Autodesk Inventor part; units mm, degrees
ref_plane "Work Plane1" through (277, 0, 0) normal (1, 0, 0) x (0, 1, 0)
ref_plane "Work Plane2" through (0, 40, 0) normal (0, 1, 0) x (-1, 0, 0)
ref_plane "XY Plane" through (0, 0, 0) normal (0, 0, 1) x (1, 0, 0)
sketch "Sketch1" plane through (0, 0, 0) normal (0, 0, 1) x (1, 0, 0)
  line L0 (955, 0) -> (955, 80)
  line L1 (0, 80) -> (0, 0)
  line L2 (277, 0) -> (277, 20)
  line L3 (277, 20) -> (733, 20)
  line L4 (733, 20) -> (733, 0)
  line L5 (277, 80) -> (277, 60)
  line L6 (277, 60) -> (733, 60)
  line L7 (733, 60) -> (733, 80)
  line L8 (0, 80) -> (955, 80)
  line L9 (427, 0) -> (427, 20)
  line L10 (583, 0) -> (583, 20)
  line L11 (0, 0) -> (955, 0)
  line L12 (277, 0) -> (733, 0)
  line L13 (733, 80) -> (277, 80)
  dimension "d0" = 955
  dimension "d1" = 80
  dimension "d2" = 277
  dimension "d3" = 20
  dimension "d4" = 456
  dimension "d5" = 150
  dimension "d6" = 150
extrude "Extrusion1" add sketch "Sketch1" along normal mid plane 5 contours L11 L4 L3 L2 L1 L8 L5 L6 L7 L0
extrude "Extrusion2" add sketch "Sketch1" along normal mid plane 10 contours L11 L10 L3 L4 | L7 L6 L5 L8 | L11 L9 L3 L10 | L11 L2 L3 L9
sketch "Sketch3" plane through (0, 0, 2.5) normal (-1, 0, 0) x (0, 0, 1)
  line L0 (-5, 0) -> (-5, 80)
  arc A0 (0, 0.0782) -> (0, 79.9218) centre (-2.5, 40) ccw
  arc A1 (0, 20.0782) -> (0, 59.9218) centre (10.4691, 40) ccw
  line L1 (0, 79.9218) -> (0, 59.9218)
  line L2 (0, 20.0782) -> (0, 0.0782)
  point P0 (-2.5, 0)
  dimension "d18" = 20
  dimension "d19" = 20
extrude "Extrusion4" add sketch "Sketch3" against normal blind 5
pattern_linear "Rectangular Pattern1" count 2 spacing 133.5 along (1, 0, 0) of "Extrusion4"
ref_plane "Work Plane1" through (277, 0, 0) normal (1, 0, 0) x (0, 1, 0)
sketch "Sketch4" plane through (277, 0, 0) normal (1, 0, 0) x (0, 1, 0)
  line L0 (80, 2.5) -> (80, -2.5)
  line L1 (80, -5) -> (80, -2.5)
  line L2 (80, -2.5) -> (80, -5)
  line L3 (80, 2.5) -> (80, -2.5)
  line L4 (80, 5) -> (80, 2.5)
  line L5 (80, 2.5) -> (80, 5)
  line L6 (0, 2.5) -> (0, -2.5)
  line L7 (0, 5) -> (0, 2.5)
  line L8 (0, 2.5) -> (0, 5)
  line L9 (0, -2.5) -> (0, 2.5)
  line L10 (0, -5) -> (0, -2.5)
  line L11 (0, -2.5) -> (0, -5)
  line L12 (80, 5) -> (60, 5)
  line L13 (60, 5) -> (80, 5)
  line L14 (20, 5) -> (0, 5)
  line L15 (0, 5) -> (20, 5)
  line L16 (60, 2.5) -> (60, 5)
  line L17 (60, 2.5) -> (60, 5)
  line L18 (20, 5) -> (20, 2.5)
  line L19 (20, 5) -> (20, 2.5)
  line L20 (78.7298, 5) -> (60, 5)
  line L21 (20, 5) -> (0.9311, 5)
  line L22 (20, 5) -> (20, 2.5)
  line L23 (60, 5) -> (60, 2.5)
  arc A0 (60, 5) -> (20, 5) centre (40, 9.7482) ccw
  line L24 (20, -2.5) -> (20, -5)
  line L25 (20, -2.5) -> (20, -5)
  line L26 (60, -5) -> (60, -2.5)
  line L27 (60, -5) -> (60, -2.5)
  arc A1 (80, 0) -> (0, 0) centre (40, 0) ccw
  line L28 (79.6863, 5) -> (60, 5)
  line L29 (20, 5) -> (0.3137, 5)
  line L30 (0.3137, 5) -> (0, 5)
  line L31 (0, 5) -> (0, 0)
  line L32 (79.6863, 5) -> (80, 5)
  line L33 (80, 5) -> (80, 0)
  point P0 (80, 5)
  point P1 (80, -5)
  point P2 (0, -5)
  point P3 (0, 5)
  dimension "d26" = 80
extrude "Extrusion5" add sketch "Sketch4" along normal blind 5 contours L12 A0 L14 A1
extrude "Extrusion6" cut sketch "Sketch4" along normal blind 500 contours A1 L6 L7 L14 | L0 A1 L12 L4
sketch "Sketch5" plane through (277, 0, -5) normal (0, -1, 0) x (1, 0, 0)
  circle A0 centre (306, 5) radius 2.5
  circle A1 centre (150, 5) radius 2.5
  point P0 (-277, 5)
  dimension "d33" = 5
  dimension "d34" = 5
extrude "Extrusion7" cut sketch "Sketch5" against normal blind 500
pattern_linear "Rectangular Pattern2" count 6 spacing 90.2 along (1, 0, 0) of "Extrusion5"
ref_plane "Work Plane2" through (0, 40, 0) normal (0, 1, 0) x (-1, 0, 0)
sketch "Sketch6" plane through (0, 40, 0) normal (0, 1, 0) x (-1, 0, 0)
  line L0 (0, -2.5) -> (0, 2.5)
  line L1 (0, 2.5) -> (0, 40)
  line L2 (0, 0) -> (100, 0)
  spline S0 degree 4 poles (0, 40) (18.8191, 40.6892) (34.5273, 38.677) (78.4206, 36.7816) (100, 0) knots 0 0 0 0 0 1 1 1 1 1
  line L3 (0, 40) -> (0, 0)
  point P0 (13.5096, 40)
  point P1 (31.8449, 38.4324)
  point P2 (61.8997, 30.8714)
  dimension "d41" = 100
revolve "Revolution1" add sketch "Sketch6" angle 360 about axis through (0, 40, 0) along (-1, 0, 0)
properties part number "konstruksi roket"
The model under review builds one solid part; all positions refer to its coordinate system, in mm. A direction names the side the tool comes from. Round coordinates to 2 decimals unless told otherwise and drop trailing zeros. Order: outer loops, then holes, each group sorted by start corner. A loop starts at its lowest first (then second) coordinate and runs counter-clockwise, first axis right, second up. Notation, with made-up numbers: (59, -33) - (69, -33) arc R20 ccw to (69, -19) - close; hole circle Ø9 at (-13.5, -0.5). An arc over 180 degrees is marked (long way). Answer in a Markdown table with one row per item.
(1) For line 1 (Z direction, x = 459.8, y = 40); line 2 (Z direction, x = 427, y = 18.5); line 3 (X direction, y = 24, z = 0), list the stretches that pass through material, from the lowest coordinate up. Write a range as from..to.
Result set:
| item | result |
|---|---|
| line 1 | z = -2.5..2.5, 30.3..40 |
| line 2 | z = -5..-2.5, 2.5..5 |
| line 3 | x = -86.81..424.5, 429.5..580.5, 585.5..955 |
(2) Clearance check with flat-ended pins moving along their axes: P1, Ø11.5, axis at y = 37.5, z = 16.5, coming from the +X side; P2, Ø2, axis at x = 727, y = 32, coming from the -Z side; P3, Ø0.8, axis at x = 447.5, z = 4, coming from the +Y side. State where each tip first meets the part, or that it passes through.
Result set:
| item | result |
|---|---|
| P1 | stops at x = 0 |
| P2 | stops at z = -2.5 |
| P3 | stops at y = 79.84 |
(3) Take a section at A-A on x = 86.5. Write out the cut boundary in (y, z).
Result set:
| item | result |
|---|---|
| outline | (0, -2.5) - (80, -2.5) - (80, 2.5) - (0, 2.5) - close |
(4) Take a section at B-B on x = 385. Write out the cut boundary in (y, z).
Result set:
| item | result |
|---|---|
| outline | (0, -5) - (20, -5) - (20, -2.5) - (60, -2.5) - (60, -5) - (80, -5) - (80, 0) arc R40 ccw to (79.69, 5) - (60, 5) - (60, 2.5) - (20, 2.5) - (20, 5) - (0.31, 5) arc R40 ccw to (0, 0) - close |
(5) Mouldability with a two-part tool opening along Z and no side actions: class faces 1 (the face through (135.965, 39.353, 35.465)), 2 (the face through (552.6, 39, 31)), 3 (the face through (502, 10, -5)) as released by +Z, released by -Z, zero draft, split by the parting line, or undercut.
Result set:
| item | result |
|---|---|
| face 1 | undercut |
| face 2 | zero draft |
| face 3 | released by -Z |
(6) Machinability: for faces 4 (the face through (279.5, 39.5, 30.3)), 5 (the face through (277, 48, 30)), 6 (the face through (0, 40, 15)), which of the approach directions +Z, -Z, +X, -X, +Y, -Y give a long, thin tool a straight path to every point of the face, cutting with its end or side? Answer none if there is none.
Result set:
| item | result |
|---|---|
| face 4 | +X |
| face 5 | +Z, +Y, -Y |
| face 6 | none |
